Input: part model. Units: mm. Frame: model coordinates. Face numbers are marked on the shaded views. A direction names the side the tool comes from. Round coordinates to 2 decimals unless told otherwise and drop trailing zeros. Loops run counter-clockwise (first coordinate to the right, second up) from the corner with the lowest first, then second, coordinate; pieces in that order, holes last.
(1) Cut plane D-D, the plane y = -7. Output: boundary loops of the cut face in (x, z).
(2) Cut plane C-C, the plane x = 2. Output: boundary loops of the cut face in (y, z), and give its area (3 significant figures).
(3) Access query for the marked faces 4, 5, 6 and 7. Directions: +Z, -Z, +X, -X, +Y, -Y. A direction counts if a zero-diameter tool reaches every point of the face in a straight line with its end or side. Return the directions, or none.
(4) First-contact query: pin 1 Ø4.5 at (x, y) = (-1.5, 41.5) entering from +Z; pin 2 Ø11 at (x, y) = (18.5, 2) entering from +Z; pin 3 Ø2 at (x, z) = (30.5, 2.5) entering from +Y. Flat tips, straight axial feed; report the tip coordinate or a pass-through.
(5) Draft query along Y for the marked faces 1, 2 and 3. Return one class per face: released by +Y, released by -Y, zero draft, split by the parting line, or undercut.
(6) Cut plane A-A, the plane y = 30. Output: boundary loops of the cut face in (x, z), and give its area (3 significant figures).
(7) Cut plane B-B, the plane z = 4.25. Output: boundary loops of the cut face in (x, y).
(8) Line query: line 1 (X direction, y = 35, z = 2.75); line 2 (X direction, y = -10, z = 5.25); line 3 (Y direction, x = 11, z = 7.25). Output: solid intervals per line, ascending.
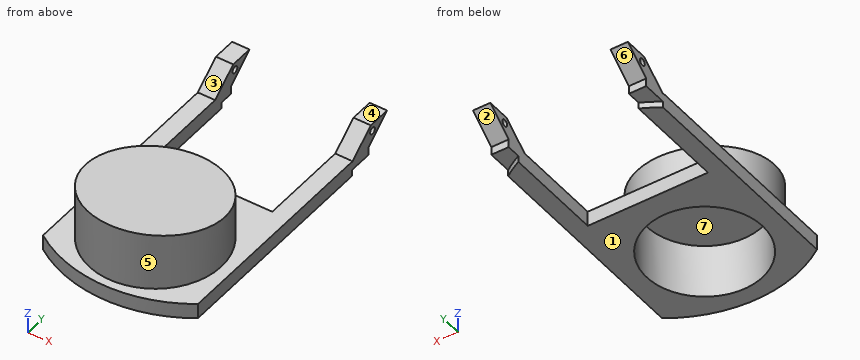
from build123d import *

# Parameters (mm, degrees)
LID_PROFILE_DEPTH           = 3.556
SKETCH2_R                   = 15.494
MOUTHPIECE_COVER_DEPTH      = 13.716
SKETCH5_R                   = 13.589
MOUTHPIECE_INSIDE_DEPTH     = 12.7
MOUTHPIECE_ANGLED_CUT_DEPTH = 31.75
LEFT_LID_HANDLE_REACH       = 54.989
RIGHT_LID_HANDLE_REACH      = 59.215
CUT_EXTRUDE1_REACH          = 61.6
SKETCH15_R                  = 0.803296428


with BuildPart() as part:
    # Sketch1 → Lid Profile (new body)
    with BuildSketch(Plane.XY):
        with BuildLine():
            Line((0, 34.499663168), (0, 21.545663168))
            Line((0, 21.545663168), (0, 11.032242365))
            Line((0, 11.032242365), (28.194, 11.032242365))
            Line((28.194, 11.032242365), (28.194, 21.545663168))
            Line((28.194, 21.545663168), (28.194, 34.499663168))
            ThreePointArc((28.194, 34.499663168), (30.270793835, 33.37243225), (32.258, 32.093865147))
            Line((32.258, 32.093865147), (32.258, -19.992239679))
            ThreePointArc((32.258, -19.992239679), (14.097, -25.699187266), (-4.064, -19.992239679))
            Line((-4.064, -19.992239679), (-4.064, 32.093865147))
            ThreePointArc((-4.064, 32.093865147), (-2.076793835, 33.37243225), (0, 34.499663168))
        make_face()
    extrude(amount=LID_PROFILE_DEPTH)

    # Sketch2 → Mouthpiece Cover (add)
    with BuildSketch(Plane.XY.offset(3.556)):
        with Locations((14.054185991, -8.173187266)):
            Circle(SKETCH2_R)
    extrude(amount=MOUTHPIECE_COVER_DEPTH)

    # Sketch5 → Mouthpiece Inside (cut)
    with BuildSketch(Plane(origin=(0, 0, 0), x_dir=(-1, 0, 0), z_dir=(0, 0, -1))):
        with Locations((-14.097, -8.173187266)):
            Circle(SKETCH5_R)
    extrude(amount=-MOUTHPIECE_INSIDE_DEPTH, mode=Mode.SUBTRACT)

    # Sketch12 → Mouthpiece Angled Cut (cut, symmetric)
    with BuildSketch(Plane(origin=(0, 0, 0), x_dir=(0, 0, -1), z_dir=(1, 0, 0))):
        Polygon((-17.272, -23.667187266), (-13.208, 7.320812734), (-17.272, 7.320812734), align=None)
    extrude(amount=MOUTHPIECE_ANGLED_CUT_DEPTH, both=True, mode=Mode.SUBTRACT)

    # Left Lid Handle: up to this face of the body (flat: up to its plane)
    left_lid_handle_end = Plane(part.part.faces().sort_by_distance((0, 22.765952767, 1.778))[0])
    # Sketch10 → Left Lid Handle (add, up to the picked face)
    with BuildSketch(Plane.ZY.offset(4.064), mode=Mode.PRIVATE) as left_lid_handle_sk1:
        Polygon((3.365795212, 32.138217174), (8.321348051, 38.515411016), (8.321348051, 43.984174588), (3.365795212, 37.782280768), (1.455115312, 37.782280768), (1.455115312, 28.897562955), (3.365795212, 28.897562955), align=None)
    left_lid_handle_tool1 = split(extrude(left_lid_handle_sk1.sketch, amount=-LEFT_LID_HANDLE_REACH, mode=Mode.PRIVATE), bisect_by=left_lid_handle_end, keep=Keep.BOTH, mode=Mode.PRIVATE)
    add(left_lid_handle_tool1.solids().sort_by(Axis((-4.064, 36.27745, 4.52617), (1, 0, 0)))[0])

    # Right Lid Handle: up to this face of the body (flat: up to its plane)
    right_lid_handle_end = Plane(part.part.faces().sort_by_distance((32.258, 6.050812734, 1.778))[0])
    # Sketch14 → Right Lid Handle (add, up to the picked face)
    with BuildSketch(Plane.ZY.offset(-28.194), mode=Mode.PRIVATE) as right_lid_handle_sk1:
        Polygon((8.321348051, 43.984174588), (8.321348051, 38.515411016), (3.365795212, 32.093865147), (3.302, 26.626354669), (1.53624021, 26.626354669), (1.455115312, 37.782280768), (3.365795212, 37.782280768), align=None)
    right_lid_handle_tool1 = split(extrude(right_lid_handle_sk1.sketch, amount=-RIGHT_LID_HANDLE_REACH, mode=Mode.PRIVATE), bisect_by=right_lid_handle_end, keep=Keep.BOTH, mode=Mode.PRIVATE)
    add(right_lid_handle_tool1.solids().sort_by(Axis((28.194, 35.592076, 4.370093), (1, 0, 0)))[0])

    # Cut-Extrude1: up to this face of the body (flat: up to its plane)
    cut_extrude1_end = Plane(part.part.faces().sort_by_distance((32.258, 11.399042149, 2.309511507))[0])
    # Sketch15 → Cut-Extrude1 (cut, up to the picked face)
    with BuildSketch(Plane.ZY.offset(4.064), mode=Mode.PRIVATE) as cut_extrude1_sk1:
        with Locations(Location((6.586858653, 39.082697022, 0), (0, 0, 270))):
            Circle(SKETCH15_R)
    cut_extrude1_tool1 = split(extrude(cut_extrude1_sk1.sketch, amount=-CUT_EXTRUDE1_REACH, mode=Mode.PRIVATE), bisect_by=cut_extrude1_end, keep=Keep.BOTH, mode=Mode.PRIVATE)
    add(cut_extrude1_tool1.solids().sort_by(Axis((-4.064, 39.082697, 6.586859), (1, 0, 0)))[0], mode=Mode.SUBTRACT)


solid = part.part
Reported:
1. outline: (-4.06, 0) - (0.56, 0) - (0.56, 12.7) - (27.64, 12.7) - (27.64, 0) - (32.26, 0) - (32.26, 3.56) - (29.5, 3.56) - (29.5, 15.09) - (-1.4, 15.09) - (-1.4, 3.56) - (-4.06, 3.56) - close
2. outline: (-23.3, 0) - (-14.36, 0) - (-14.36, 12.7) - (-1.98, 12.7) - (-1.98, 0) - (11.03, 0) - (11.03, 3.56) - (1.56, 3.56) - (1.56, 13.96) - (-17.91, 16.52) - (-17.91, 3.56) - (-23.3, 3.56) - close
2. area: 192 mm2
3. face 4: +Z, +X, -X, +Y
3. face 5: +Z
3. face 6: -Z, +X, -X, +Y
3. face 7: -Z
4. pin 1: stops at z = 8.32
4. pin 2: stops at z = 14.63
4. pin 3: stops at y = 37.95
5. face 1: zero draft
5. face 2: released by +Y
5. face 3: undercut
6. outline: (-4.06, 0) - (0, 0) - (0, 3.56) - (-4.06, 3.56) - close; (28.19, 0) - (32.26, 0) - (32.26, 3.56) - (28.19, 3.56) - close
6. area: 28.9 mm2
7. outline: (-4.06, 33.28) - (0, 33.28) - (0, 38.89) - (-4.06, 38.89) - close; circle Ø30.99 at (14.05, -8.17); (28.19, 33.24) - (32.26, 33.24) - (32.26, 38.89) - (28.19, 38.89) - close; hole circle Ø27.18 at (14.1, -8.17)
8. line 1: x = -4.06 to 0, 28.19 to 32.26
8. line 2: x = -1.33 to 0.63, 27.56 to 29.44
8. line 3: y = -23.36 to -21.4, 5.06 to 7.02
